Can you work these out from the model? Positions are in its coordinate system, mm. A direction names the side the tool comes from. Give positions to 0.01 mm unless a question says otherwise; leave off trailing zeros. Order: outer loops, then holes, each group sorted by start corner. A loop starts at its lowest first (then second) coordinate and runs counter-clockwise, first axis right, second up. Notation, with made-up numbers: (55, 16.5) -> (74, 16.5) arc R22 cw to (74, 42.5) -> close; hole circle Ø6 at (-1.75, 19.5). An arc over 180 degrees is marked (long way). Answer as CSV lines item,"result".
```python
from build123d import *

# Parameters (mm, degrees)
SKETCH1_W           = 250
SKETCH1_H           = 200
SKETCH1_W_2         = 230
SKETCH1_H_2         = 184
BOSS_EXTRUDE1_DEPTH = 125
SKETCH2_W           = 250
SKETCH2_H           = 200
BOSS_EXTRUDE2_DEPTH = 5
SKETCH3_R           = 2.5
CUT_EXTRUDE1_DEPTH  = 5
SKETCH4_W           = 56.888032222
SKETCH4_H           = 3
CUT_EXTRUDE2_DEPTH  = 10
SKETCH5_R           = 2.28
CUT_EXTRUDE3_DEPTH  = 10
SKETCH6_W           = 51.923491606
SKETCH6_H           = 2.813206455
SKETCH6_W_2         = 1.706106107
SKETCH6_H_2         = 39.950466237
SKETCH6_W_3         = 35.31144106
SKETCH6_H_3         = 3.552801372
CUT_EXTRUDE4_DEPTH  = 10


with BuildPart() as part:
    # Sketch1 → Boss-Extrude1 (new body)
    with BuildSketch(Plane(origin=(0, 0, 0), x_dir=(1, 0, 0), z_dir=(0, 1, 0))):
        Rectangle(SKETCH1_W, SKETCH1_H)
        Rectangle(SKETCH1_W_2, SKETCH1_H_2, mode=Mode.SUBTRACT)
    extrude(amount=BOSS_EXTRUDE1_DEPTH)

    # Sketch2 → Boss-Extrude2 (add)
    with BuildSketch(Plane(origin=(0, 0, 0), x_dir=(1, 0, 0), z_dir=(0, 1, 0))):
        Rectangle(SKETCH2_W, SKETCH2_H)
    extrude(amount=-BOSS_EXTRUDE2_DEPTH)

    # Sketch3 → Cut-Extrude1 (cut)
    with BuildSketch(Plane(origin=(0, 125, 0), x_dir=(1, 0, 0), z_dir=(0, 1, 0))):
        with Locations(Location((-119.900696791, -94.21890742, 0), (0, 0, 270))):
            Circle(SKETCH3_R)
        with Locations(Location((-119.900696791, 94.21890742, 0), (0, 0, 90))):
            Circle(SKETCH3_R)
        with Locations(Location((119.900696791, 94.21890742, 0), (0, 0, 270))):
            Circle(SKETCH3_R)
        with Locations(Location((119.900696791, -94.21890742, 0), (0, 0, 90))):
            Circle(SKETCH3_R)
    extrude(amount=-CUT_EXTRUDE1_DEPTH, mode=Mode.SUBTRACT)

    # Sketch4 → Cut-Extrude2 (cut)
    with BuildSketch(Plane.XY.offset(100)):
        with Locations((-78.091753323, 108.422214629)):
            Rectangle(SKETCH4_W, SKETCH4_H)
        with Locations((-78.091753323, 101.422214629)):
            Rectangle(SKETCH4_W, SKETCH4_H)
        with Locations((-78.091753323, 94.422214629)):
            Rectangle(SKETCH4_W, SKETCH4_H)
    extrude(amount=-CUT_EXTRUDE2_DEPTH, mode=Mode.SUBTRACT)

    # Sketch5 → Cut-Extrude3 (cut)
    with BuildSketch(Plane(origin=(0, 0, -100), x_dir=(-1, 0, 0), z_dir=(0, 0, -1))):
        with Locations((-42.656938609, 32.257458939)):
            Circle(SKETCH5_R)
        with Locations((-113.658122402, 103.257458939)):
            Circle(SKETCH5_R)
        with Locations(Location((-42.656938609, 103.257458939, 0), (0, 0, 180))):
            Circle(SKETCH5_R)
        with Locations(Location((-113.658122402, 32.257458939, 0), (0, 0, 126.053669341))):
            Circle(SKETCH5_R)
    extrude(amount=-CUT_EXTRUDE3_DEPTH, mode=Mode.SUBTRACT)

    # Sketch6 → Cut-Extrude4 (cut)
    with BuildSketch(Plane(origin=(0, 0, -100), x_dir=(-1, 0, 0), z_dir=(0, 0, -1))):
        with Locations((-78.080252777, 90.048098673)):
            Rectangle(SKETCH6_W, SKETCH6_H)
        with Locations((-78.080252777, 95.048098673)):
            Rectangle(SKETCH6_W, SKETCH6_H)
        with Locations((-78.080252777, 85.048098673)):
            Rectangle(SKETCH6_W, SKETCH6_H)
        with Locations((-78.080252777, 80.048098673)):
            Rectangle(SKETCH6_W, SKETCH6_H)
        with Locations((-78.080252777, 75.048098673)):
            Rectangle(SKETCH6_W, SKETCH6_H)
        with Locations((-78.080252777, 70.048098673)):
            Rectangle(SKETCH6_W, SKETCH6_H)
        with Locations((-78.080252777, 65.048098673)):
            Rectangle(SKETCH6_W, SKETCH6_H)
        with Locations((-78.080252777, 60.048098673)):
            Rectangle(SKETCH6_W, SKETCH6_H)
        with Locations((-78.080252777, 55.048098673)):
            Rectangle(SKETCH6_W, SKETCH6_H)
        with Locations((-78.080252777, 50.048098673)):
            Rectangle(SKETCH6_W, SKETCH6_H)
        with Locations((-78.080252777, 45.048098673)):
            Rectangle(SKETCH6_W, SKETCH6_H)
        with Locations((-78.080252777, 40.048098673)):
            Rectangle(SKETCH6_W, SKETCH6_H)
        with Locations((-109.706066926, 66.479468782)):
            Rectangle(SKETCH6_W_2, SKETCH6_H_2)
        with Locations((-46.608994087, 66.479468782)):
            Rectangle(SKETCH6_W_2, SKETCH6_H_2)
        with Locations((-76.965618839, 101.05962005)):
            Rectangle(SKETCH6_W_3, SKETCH6_H_3)
        with Locations((-76.965618839, 34.455297829)):
            Rectangle(SKETCH6_W_3, SKETCH6_H_3)
    extrude(amount=-CUT_EXTRUDE4_DEPTH, mode=Mode.SUBTRACT)


solid = part.part
```
Item 1: Imagine slicing it at C-C, the plane x = -29. Please give me the cut outline in (y, z).
Numbers:
outline,"(-5, -100) -> (125, -100) -> (125, -92) -> (0, -92) -> (0, 92) -> (125, 92) -> (125, 100) -> (-5, 100) -> close"
Item 2: For faces 3 (the flat face through (-78, 102.922, 96)), 4 (the flat face through (-115, 62, 1)), 5 (the flat face through (78, 53.641, -96)), which set-ups out of +Z, -Z, +X, -X, +Y, -Y let a thin tool reach every point of the face, with its end or its side?
Numbers:
face 3,"+Z"
face 4,"+Y"
face 5,"-Z"
Item 3: Imagine slicing it at B-B, the plane y = 8. Please give me the cut outline in (x, z).
Numbers:
outline,"(-125, -100) -> (125, -100) -> (125, 100) -> (-125, 100) -> close; hole (-115, -92) -> (115, -92) -> (115, 92) -> (-115, 92) -> close"
Item 4: We'd pull the mould along X, two halves only. Please class faces 1 (the flat face through (-125, 61, 1)), 2 (the flat face through (78, 58.641, -96)): released by +X, released by -X, zero draft, split by the parting line, or undercut.
Numbers:
face 1,"released by -X"
face 2,"undercut"
Item 5: Imagine slicing it at D-D, the plane z = 73.5. Please give me the cut outline in (x, y).
Numbers:
outline,"(-125, -5) -> (125, -5) -> (125, 125) -> (115, 125) -> (115, 0) -> (-115, 0) -> (-115, 125) -> (-125, 125) -> close"
Item 6: Imagine slicing it at A-A, the plane x = -102. Please give me the cut outline in (y, z).
Numbers:
outline,"(-5, -100) -> (125, -100) -> (125, -92) -> (0, -92) -> (0, 92) -> (92.92, 92) -> (92.92, 100) -> (-5, 100) -> close; (95.92, 92) -> (99.92, 92) -> (99.92, 100) -> (95.92, 100) -> close; (102.92, 92) -> (106.92, 92) -> (106.92, 100) -> (102.92, 100) -> close; (109.92, 92) -> (125, 92) -> (125, 100) -> (109.92, 100) -> close"
Item 7: For pin 1 (6 mm diameter, centred on x = 12, z = -66.5, fed in from +Y); pin 2 (6.5 mm diameter, centred on x = 119.9, z = 94.22, fed in from +Y), each with a flat end and sliding along its axis, tell me the tip position at first contact or that it passes through.
Numbers:
pin 1,"stops at y = 0"
pin 2,"stops at y = 125"
Item 8: Please list where these lines run through material, in increasing order: line 1 along X through (y, z) = (79, -47); line 2 along Z through (x, y) = (-54, 83.5); line 3 along Y through (x, z) = (3, -91).
Numbers:
line 1,"x = -125 to -115, 115 to 125"
line 2,"z = -100 to -92, 92 to 100"
line 3,"y = -5 to 0"
